The listing builds one solid part. Answer for the finished solid, in the listing's coordinates (mm). A direction names the side the tool comes from. Round coordinates to 2 decimals unless told otherwise and drop trailing zeros. Loops run counter-clockwise (first coordinate to the right, second up) from the corner with the lowest first, then second, coordinate; pieces in that order, holes last. Notation, with made-up numbers: (69, 35.5) - (77, 35.5) arc R31 ccw to (77, 67.5) - close; hole circle Ø5 at (85, -22.5). An arc over 180 degrees is marked (long way). One line per item, written item: value.
Autodesk Inventor part; units mm, degrees
sketch "Sketch1" plane through (0, 0, 0) normal (0, 0, 1) x (1, 0, 0)
  line L0 (0, 0) -> (0, 40)
  line L1 (0, 40) -> (30, 40)
  line L2 (30, 40) -> (30, 37)
  line L3 (30, 37) -> (3, 37)
  line L4 (3, 37) -> (3, 0)
  line L5 (3, 0) -> (0, 0)
extrude "Extrusion1" add sketch "Sketch1" along normal blind 30
sketch "Sketch2" plane through (3, 0, 0) normal (1, 0, 0) x (0, 0, -1)
  line L0 (-30, 37) -> (-30, 40)
  line L1 (-30, 40) -> (-20, 40)
  line L2 (0, 40) -> (-30, 40)
  line L3 (0, 0) -> (-30, 0)
  line L4 (-20, 0) -> (-10, 0)
  line L5 (0, 37) -> (-30, 37)
  circle A0 centre (-20, 32) radius 1.5
  circle A1 centre (-20, 5) radius 1.5
  circle A2 centre (-10, 20) radius 1.5
extrude "Extrusion2" cut sketch "Sketch2" against normal blind 30
sketch "Sketch3" plane through (0, 40, 0) normal (0, 1, 0) x (1, 0, 0)
  line L0 (0, 0) -> (0, -30)
  line L1 (3, 0) -> (30, 0)
  line L2 (3, -30) -> (30, -30)
  circle A0 centre (15, -15) radius 1.5
extrude "Extrusion3" cut sketch "Sketch3" against normal blind 30
sketch "Sketch4" plane through (0, 40, 0) normal (0, 1, 0) x (1, 0, 0)
  circle A0 centre (15, -15) radius 1.5
  circle A1 centre (15, -15) radius 1.5
  point P0 (0, 0)
extrude "Extrusion4" add sketch "Sketch4" against normal blind 3
sketch "Sketch5" plane through (0, 40, 0) normal (0, 1, 0) x (1, 0, 0)
  point P0 (0, 0)
sketch "Sketch6" plane through (0, 40, 0) normal (0, 1, 0) x (1, 0, 0)
  line L0 (3, -30) -> (30, -30)
  circle A0 centre (15, -22.5) radius 1.5
  circle A1 centre (15, -7.5) radius 1.5
  point P0 (0, 0)
extrude "Extrusion5" cut sketch "Sketch6" against normal blind 3
properties part number "T_shape"
1) A cutting plane is placed at D-D on y = 32. Give the vertices of the cut face in (x, z).
Final values:
outline: (0, 0) - (3, 0) - (3, 18.5) - (0, 18.5) - close; (0, 21.5) - (3, 21.5) - (3, 30) - (0, 30) - close
2) For faces 4 (the flat face through (17, 37, 15)), 5 (the cylindrical face through (1.52, 21.01, 11.11)), determine the directions among +Z, -Z, +X, -X, +Y, -Y from which every point of the face is accessible in a straight line to the end or side of a thin tool.
Final values:
face 4: +Z, -Z, +X, -Y
face 5: +X, -X
3) For a pull along X with two mould halves and no side action, classify faces 1 (the cylindrical face through (13.8, 38.5, 8.4)), 2 (the flat face through (30, 39, 15)), 3 (the flat face through (15, 40, 15)) as released by +X, released by -X, zero draft, split by the parting line, or undercut.
Final values:
face 1: undercut
face 2: released by +X
face 3: zero draft
4) This flat-tipped pin is pushed along its axis until it touches: pin 1 Ø2.5 at (y, z) = (20, 10) entering from -X. Where does it stop, or does it pass through?
Final values:
pin 1: through
5) A cutting plane is placed at B-B on x = 15. Give the vertices of the cut face in (y, z).
Final values:
outline: (37, 0) - (40, 0) - (40, 6) - (37, 6) - close; (37, 9) - (40, 9) - (40, 21) - (37, 21) - close; (37, 24) - (40, 24) - (40, 30) - (37, 30) - close
6) Consider L1, parallel to Z at x = 15, y = 38.55; L2, parallel to Y at x = 1.75, z = 20; L3, parallel to X at y = 38.8, z = 7.5. Determine where each line is inside the solid, lowest interval first.
Final values:
L1: 0 to 6, 9 to 21, 24 to 30
L2: 0 to 3.5, 6.5 to 30.5, 33.5 to 40
L3: 0 to 13.5, 16.5 to 30
7) A cutting plane is placed at A-A on z = 20. Give the vertices of the cut face in (x, y).
Final values:
outline: (0, 0) - (3, 0) - (3, 3.5) - (0, 3.5) - close; (0, 6.5) - (3, 6.5) - (3, 30.5) - (0, 30.5) - close; (0, 33.5) - (3, 33.5) - (3, 37) - (30, 37) - (30, 40) - (0, 40) - close
8) A cutting plane is placed at C-C on z = 10. Give the vertices of the cut face in (x, y).
Final values:
outline: (0, 0) - (3, 0) - (3, 18.5) - (0, 18.5) - close; (0, 21.5) - (3, 21.5) - (3, 37) - (30, 37) - (30, 40) - (0, 40) - close
